The drawing under review shows one solid part. Ordinate dimensions are in mm from its lowest x, y, z. Round coordinates to 2 decimals unless told otherwise and drop trailing zeros. Write each loop counter-clockwise with the first axis right and the second up, starting at its lowest first coordinate (ties: lowest second). Pieces come first, ordered by that corner, then holes. Notation, with made-up numbers: (43, -22) -> (73, -22) arc R8 cw to (73, -13) -> close; hole circle Ø5 at (50, -32). An arc over 180 degrees is marked (long way). Write item = value, one per line. Start each with the question number.
Item 1: Add section D-D, the plane y = 0.75. State the section outline as (x, z) points (3 decimals), then the cut area to 3 significant figures.
Item 2: Add section A-A, the plane z = 2.5. State the section outline as (x, y) points.
Item 3: Add section B-B, the plane y = 4. State the section outline as (x, z) points (3 decimals), then the cut area to 3 significant figures.
Item 4: For pin 1 Ø1 at (x, y) = (32.5, 3.5) entering from -Z, flat-tipped, find the tip position at first contact; note if it passes through.
Item 5: Add section C-C, the plane x = 45.72. State the section outline as (y, z) points (3 decimals).
Item 6: To check wall thickness, follow L1, parallel to X at y = 2.25, z = 2.25; L2, parallel to X at y = 4.5, z = 3.5; L3, parallel to Z at x = 35.5, y = 3. State the ranges of each line that lie inside material, in increasing order.
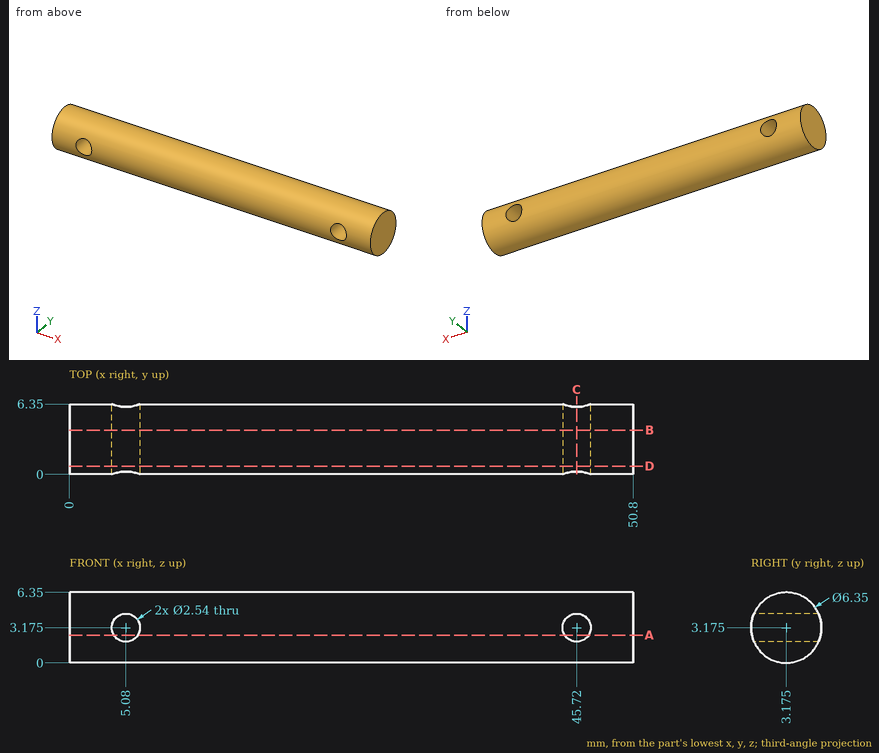
Result set:
q1.outline = (0, 1.126) -> (50.8, 1.126) -> (50.8, 5.224) -> (0, 5.224) -> close; hole circle Ø2.54 at (5.08, 3.175); hole circle Ø2.54 at (45.72, 3.175)
q1.area = 198 mm²
q2.outline = (0, 0.07) -> (4, 0.07) -> (4, 6.28) -> (0, 6.28) -> close; (6.16, 0.07) -> (44.64, 0.07) -> (44.64, 6.28) -> (6.16, 6.28) -> close; (46.8, 0.07) -> (50.8, 0.07) -> (50.8, 6.28) -> (46.8, 6.28) -> close
q3.outline = (0, 0.109) -> (50.8, 0.109) -> (50.8, 6.241) -> (0, 6.241) -> close; hole circle Ø2.54 at (5.08, 3.175); hole circle Ø2.54 at (45.72, 3.175)
q3.area = 301 mm²
q4.pin_1 = 0
q5.outline = (0.265, 1.905) arc R3.175 ccw to (6.085, 1.905) -> close; (0.265, 4.445) -> (6.085, 4.445) arc R3.175 ccw to start
q6.L1 = 0 to 4.21, 5.95 to 44.85, 46.59 to 50.8
q6.L2 = 0 to 3.85, 6.31 to 44.49, 46.95 to 50.8
q6.L3 = 0 to 6.35
